Autodesk Inventor part; units mm, degrees
ref_plane "YZ Plane" through (0, 0, 0) normal (1, 0, 0) x (0, 1, 0)
ref_plane "XZ Plane" through (0, 0, 0) normal (0, 1, 0) x (-1, 0, 0)
ref_plane "XY Plane" through (0, 0, 0) normal (0, 0, 1) x (1, 0, 0)
sketch "Sketch1" plane through (0, 0, 0) normal (0, 1, 0) x (-1, 0, 0)
  circle A0 centre (0, 0) radius 8
  dimension "d0" = 16
extrude "Extrusion1" add sketch "Sketch1" along normal blind 7.5
sketch "Sketch2" plane through (0, 7.5, 0) normal (0, 1, 0) x (1, 0, 0)
  circle A0 centre (0, 0) radius 8
  line L0 (8, 0) -> (-8, 0)
  line L1 (0, -8) -> (0, 8)
hole "Hole1" at (0, 7.5, 0) direction (0, -1, 0) diameter 10 end through all
sketch "Sketch3" plane through (0, 0, 0) normal (0, -1, 0) x (1, 0, 0)
  circle A0 centre (0, 0) radius 8
extrude "Extrusion2" add sketch "Sketch3" along normal blind 1
properties part number "Drukhulse"
For this review, take the finished solid that the model builds, in its own axes (mm). A direction names the side the tool comes from. Round coordinates to 2 decimals unless told otherwise and drop trailing zeros. Loops run counter-clockwise (first coordinate to the right, second up) from the corner with the lowest first, then second, coordinate; pieces in that order, holes last.
Q1. Add section A-A on x = 0. Write out the cut boundary in (y, z), plus the area to 3 significant figures.
Result sheet:
outline: (-1, -8) - (7.5, -8) - (7.5, -5) - (0, -5) - (0, 5) - (7.5, 5) - (7.5, 8) - (-1, 8) - close
area: 61.0 mm2
Q2. Mouldability with a two-part tool opening along X and no side actions: class faces 3 (the face through (4.88, 3.7, -1.08)), 4 (the face through (0, -1, 0)) as +X half, -X half, draft (parallel to the pull), parting line (faces both ways), or undercut.
Result sheet:
face 3: undercut
face 4: draft
Q3. Insertion check: pin 1 Ø3 at (x, z) = (0.5, 1.5) entering from +Y. The pin has a flat end and moves straight along its axis. Give the tip position at first contact, or say it passes through.
Result sheet:
pin 1: stops at y = 0
Q4. Add section C-C on y = 3.75. Write out the cut boundary in (x, z).
Result sheet:
outline: circle Ø16 at (0, 0); hole circle Ø10 at (0, 0)
Q5. Add section D-D on z = -7. Write out the cut boundary in (x, y), plus the area to 3 significant figures.
Result sheet:
outline: (-3.87, -1) - (3.87, -1) - (3.87, 7.5) - (-3.87, 7.5) - close
area: 65.8 mm2
Q6. Add section B-B on z = -1. Write out the cut boundary in (x, y), plus the area to 3 significant figures.
Result sheet:
outline: (-7.94, -1) - (7.94, -1) - (7.94, 7.5) - (4.9, 7.5) - (4.9, 0) - (-4.9, 0) - (-4.9, 7.5) - (-7.94, 7.5) - close
area: 61.4 mm2
Q7. To check wall thickness, follow line 1 along Z through (x, y) = (0, 5.5); line 2 along X through (y, z) = (3.5, 1.75). State the ranges of each line that lie inside material, in increasing order.
Result sheet:
line 1: z = -8 to -5, 5 to 8
line 2: x = -7.81 to -4.68, 4.68 to 7.81
Q8. Machinability: for faces 1 (the face through (0, 0, 0)), 2 (the face through (0.1, 7.5, -5.2)), which of the approach directions +Z, -Z, +X, -X, +Y, -Y give a long, thin tool a straight path to every point of the face, cutting with its end or side? Answer none if there is none.
Result sheet:
face 1: +Y
face 2: +Z, -Z, +X, -X, +Y
